Autodesk Inventor part; units mm, degrees
ref_plane "YZ Plane" through (0, 0, 0) normal (1, 0, 0) x (0, 1, 0)
ref_plane "XZ Plane" through (0, 0, 0) normal (0, 1, 0) x (-1, 0, 0)
ref_plane "XY Plane" through (0, 0, 0) normal (0, 0, 1) x (1, 0, 0)
sketch "Szkic1" plane through (0, 0, 0) normal (0, 0, 1) x (1, 0, 0)
  line L0 (-9.6941, 6.7253) -> (-9.6941, -58.2747)
  line L1 (-9.6941, 6.7253) -> (55.3059, 6.7253)
  line L2 (55.3059, 6.7253) -> (55.3059, -13.2747)
  line L3 (55.3059, -13.2747) -> (10.3059, -13.2747)
  line L4 (10.3059, -13.2747) -> (10.3059, -58.2747)
  line L5 (10.3059, -58.2747) -> (-9.6941, -58.2747)
  point P0 (0, 0)
  point P1 (0.3059, -48.2747)
  point P2 (0.3059, -25.7747)
  point P3 (0.3059, -3.2747)
  point P4 (45.3059, -3.2747)
  point P5 (22.8059, -3.2747)
  dimension "d0" = 65
  dimension "d1" = 65
  dimension "d2" = 20
  dimension "d4" = 10
  dimension "d5" = 10
  dimension "d6" = 20
  dimension "d7" = 10
  dimension "d8" = 10
  dimension "d9" = 10
  dimension "d10" = 22.5
  dimension "d11" = 22.5
  dimension "d12" = 10
  dimension "d13" = 10
  dimension "d14" = 10
extrude "Wyciągnięcie proste1" add sketch "Szkic1" along normal blind 3
hole "Otwór1" at (0.3059, -48.2747, 0) at (0.3059, -25.7747, 0) at (0.3059, -3.2747, 0) at (45.3059, -3.2747, 0) at (22.8059, -3.2747, 0) direction (0, 0, 1) diameter 5 end through all
fillet "Zaokrąglenie1" radius 4 5 edges at (-9.6941, 6.7253, 1.5) (55.3059, 6.7253, 1.5) (55.3059, -13.2747, 1.5) (10.3059, -58.2747, 1.5) (-9.6941, -58.2747, 1.5)
fillet "Zaokrąglenie2" radius 20 1 edges at (10.3059, -13.2747, 1.5)
properties part number "LC_ALU_3mm_Top_Beam_Mounting_Bracket" material "Aluminium 6061-AHC"
The listing builds one solid part. Answer for the finished solid, in the listing's coordinates (mm). A direction names the side the tool comes from. Coordinates: 2 decimals unless noted, no trailing zeros. Write each loop counter-clockwise with the first axis right and the second up, starting at its lowest first coordinate (ties: lowest second). Pieces come first, ordered by that corner, then holes. Notation, with made-up numbers: (84.25, 21.25) - (95.25, 21.25) arc R22 ccw to (95.25, 29.25) - close; hole circle Ø3 at (-31.5, -29.75). An arc over 180 degrees is marked (long way). Return JSON: item names as keys, results as strings.
1. For a pull along Y with two mould halves and no side action, classify faces 1 (the face through (9.103, -57.134, 1.521)), 2 (the face through (54.17, 5.52, 1.52)), 3 (the face through (-9.694, -25, 1)), 4 (the face through (20.327, -3.6, 1.521)) as +Y half, -Y half, draft (parallel to the pull), parting line (faces both ways), or undercut.
Final values:
{"face 1": "-Y half", "face 2": "+Y half", "face 3": "draft", "face 4": "undercut"}
2. The part is cut by section B-B on x = 21.5. Determine the outline of the cut face in (y, z), then the cut area to 3 significant figures.
Final values:
{"outline": "(-15.32, 0) - (-5.41, 0) - (-5.41, 3) - (-15.32, 3) - close; (-1.14, 0) - (6.73, 0) - (6.73, 3) - (-1.14, 3) - close", "area": "53.3 mm^2"}
3. The part is cut by section A-A on y = -2.5. Determine the outline of the cut face in (x, z), then the cut area to 3 significant figures.
Final values:
{"outline": "(-9.69, 0) - (-2.07, 0) - (-2.07, 3) - (-9.69, 3) - close; (2.68, 0) - (20.43, 0) - (20.43, 3) - (2.68, 3) - close; (25.18, 0) - (42.93, 0) - (42.93, 3) - (25.18, 3) - close; (47.68, 0) - (55.31, 0) - (55.31, 3) - (47.68, 3) - close", "area": "152 mm^2"}
4. Which of the six approach directions +Z, -Z, +X, -X, +Y, -Y give full straight-line access (tool end or side, diameter ignored) to faces 5 (the face through (41, -13.275, 1)), 6 (the face through (-8.491, 5.585, 1.521))?
Final values:
{"face 5": "+Z, -Z, +X, -Y", "face 6": "+Z, -Z, -X, +Y"}
5. The part is cut by section D-D on y = -48.5. Determine the outline of the cut face in (x, z), then the cut area to 3 significant figures.
Final values:
{"outline": "(-9.69, 0) - (-2.18, 0) - (-2.18, 3) - (-9.69, 3) - close; (2.8, 0) - (10.31, 0) - (10.31, 3) - (2.8, 3) - close", "area": "45.1 mm^2"}
6. The part is cut by section C-C on z = 1.25. Determine the outline of the cut face in (x, y).
Final values:
{"outline": "(-9.69, -54.27) arc R4 ccw to (-5.69, -58.27) - (6.31, -58.27) arc R4 ccw to (10.31, -54.27) - (10.31, -33.27) arc R20 cw to (30.31, -13.27) - (51.31, -13.27) arc R4 ccw to (55.31, -9.27) - (55.31, 2.73) arc R4 ccw to (51.31, 6.73) - (-5.69, 6.73) arc R4 ccw to (-9.69, 2.73) - close; hole circle Ø5 at (0.31, -48.27); hole circle Ø5 at (0.31, -25.77); hole circle Ø5 at (0.31, -3.27); hole circle Ø5 at (22.81, -3.27); hole circle Ø5 at (45.31, -3.27)"}
7. Consider line 1 along X through (y, z) = (-3.5, 0.65); line 2 along Y through (x, z) = (45, 0.85); line 3 along X through (y, z) = (-4, 1.65). Determine where each line is inside the solid, lowest interval first.
Final values:
{"line 1": "-9.69 to -2.18, 2.8 to 20.32, 25.3 to 42.82, 47.8 to 55.31", "line 2": "-13.27 to -5.76, -0.79 to 6.73", "line 3": "-9.69 to -2.09, 2.7 to 20.41, 25.2 to 42.91, 47.7 to 55.31"}
8. Each of these flat-tipped pins is pushed along its axis until it touches: pin 1 Ø1 at (x, z) = (46.5, 1.5) entering from -Y; pin 2 Ø4 at (x, y) = (0.31, -3.27) entering from +Z. Where does it stop, or does it pass through?
Final values:
{"pin 1": "y = -13.27", "pin 2": "through"}
